```python
from build123d import *
from build123d.topology import SkipClean

# Parameters (mm, degrees)
CROQUIS1_R              = 25
SALIENTE_EXTRUIR1_DEPTH = 50
CORTAR_EXTRUIR1_DEPTH   = 50
MATRIZC2_COUNT          = 3
CROQUIS4_R              = 4
CROQUIS4_R_2            = 2
SALIENTE_EXTRUIR2_DEPTH = 15
CROQUIS4_2_R            = 2
CORTAR_EXTRUIR3_DEPTH   = 20
MATRIZC3_COUNT          = 3
MATRIZC4_COUNT          = 3
CROQUIS4_3_R            = 4
CROQUIS4_3_R_2          = 2
CORTAR_EXTRUIR4_DEPTH   = 2.5
MATRIZC5_COUNT          = 3


with BuildPart() as part:
    # Croquis1 → Saliente-Extruir1 (new body)
    with BuildSketch(Plane.XY):
        Circle(CROQUIS1_R)
    extrude(amount=SALIENTE_EXTRUIR1_DEPTH)

    # Croquis2 → Cortar-Extruir1 (cut)
    with BuildSketch(Plane(origin=(0, 0, 0), x_dir=(-1, 0, 0), z_dir=(0, 0, -1))):
        with BuildLine():
            Line((-15, 20), (15, 20))
            ThreePointArc((15, 20), (0, 25), (-15, 20))
        make_face()
    cortar_extruir1 = extrude(amount=-CORTAR_EXTRUIR1_DEPTH, mode=Mode.SUBTRACT)

    # MatrizC2: Cortar-Extruir1 ×3 about axis
    matrizc2_axis = Axis((0, 0, 0), (0, 0, 1))
    for i in range(1, MATRIZC2_COUNT):
        add(cortar_extruir1.rotate(matrizc2_axis, i * 360 / MATRIZC2_COUNT), mode=Mode.SUBTRACT)

    # Croquis4 → Saliente-Extruir2 (add, symmetric)
    with BuildSketch(Plane(origin=(0, 0, 0), x_dir=(0, 0, -1), z_dir=(1, 0, 0))):
        with Locations((0, 20)):
            Circle(CROQUIS4_R)
        with Locations((0, 20)):
            Circle(CROQUIS4_R_2, mode=Mode.SUBTRACT)
    saliente_extruir2 = extrude(amount=SALIENTE_EXTRUIR2_DEPTH, both=True)

    # Croquis4<2> → Cortar-Extruir3 (cut, symmetric)
    with SkipClean():  # the faces are left unmerged after this step: merging them gives an invalid solid
        with BuildSketch(Plane(origin=(0, 0, 0), x_dir=(0, 0, -1), z_dir=(1, 0, 0))):
            with Locations(Location((0, 20, 0), (0, 0, 180))):
                Circle(CROQUIS4_2_R)
        cortar_extruir3 = extrude(amount=CORTAR_EXTRUIR3_DEPTH, both=True, mode=Mode.SUBTRACT)

    # MatrizC3: Saliente-Extruir2 ×3 about axis
    with SkipClean():  # the faces are left unmerged after this step: merging them gives an invalid solid
        matrizc3_axis = Axis((0, 0, 0), (0, 0, 1))
        for i in range(1, MATRIZC3_COUNT):
            add(saliente_extruir2.rotate(matrizc3_axis, i * 360 / MATRIZC3_COUNT))

    # MatrizC4: Cortar-Extruir3 ×3 about axis
    with SkipClean():  # the faces are left unmerged after this step: merging them gives an invalid solid
        matrizc4_axis = Axis((0, 0, 50), (0, 0, -1))
        for i in range(1, MATRIZC4_COUNT):
            add(cortar_extruir3.rotate(matrizc4_axis, i * 360 / MATRIZC4_COUNT), mode=Mode.SUBTRACT)

    # Croquis4<3> → Cortar-Extruir4 (cut, symmetric)
    with BuildSketch(Plane(origin=(0, 0, 0), x_dir=(0, 0, -1), z_dir=(1, 0, 0))):
        with Locations((0, 20)):
            Circle(CROQUIS4_3_R)
        with Locations(Location((0, 20, 0), (0, 0, 180))):
            Circle(CROQUIS4_3_R_2, mode=Mode.SUBTRACT)
    cortar_extruir4 = extrude(amount=CORTAR_EXTRUIR4_DEPTH, both=True, mode=Mode.SUBTRACT)

    # MatrizC5: Cortar-Extruir4 ×3 about axis
    matrizc5_axis = Axis((0, 0, 0), (0, 0, 1))
    for i in range(1, MATRIZC5_COUNT):
        add(cortar_extruir4.rotate(matrizc5_axis, i * 360 / MATRIZC5_COUNT), mode=Mode.SUBTRACT)


solid = part.part
```
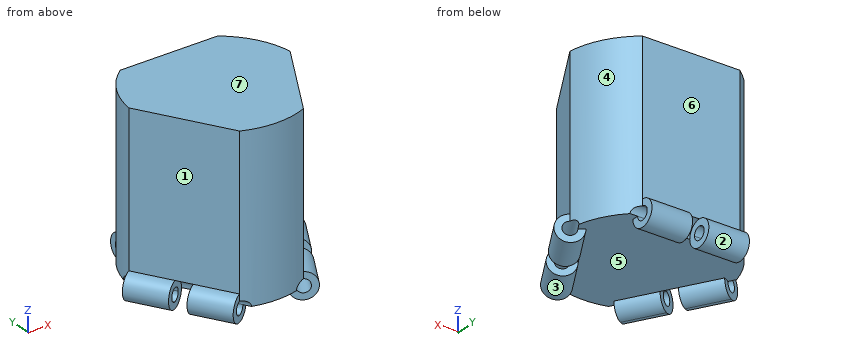
Build history of the part. All positions in model axes, mm. Face numbers are marked on the shaded views. A direction names the side the tool comes from. Round coordinates to 2 decimals unless told otherwise and drop trailing zeros. Order: outer loops, then holes, each group sorted by start corner. A loop starts at its lowest first (then second) coordinate and runs counter-clockwise, first axis right, second up. Notation, with made-up numbers: (-6.5, -30.5) -> (7.5, -30.5) arc R28 ccw to (7.5, 8.5) -> close; hole circle Ø7 at (-33, 64.5). An arc over 180 degrees is marked (long way). Answer in a Markdown table with one row per item.
1) Mould opens along X. For the marked faces 1, 2, 3 and 4 say: released by +X, released by -X, zero draft, split by the parting line, or undercut.
Values:
| item | result |
|---|---|
| face 1 | released by -X |
| face 2 | zero draft |
| face 3 | undercut |
| face 4 | released by +X |
2) Wall check: L1, parallel to Z at x = 1, y = -21.5; L2, parallel to X at y = 13, z = 30.5; L3, parallel to Y at x = 6, z = 27. Give the ranges that are in metal, low to high.
Values:
| item | result |
|---|---|
| L1 | 0 to 50 |
| L2 | -21.35 to 21.35 |
| L3 | -24.27 to 20 |
3) Band-saw the part on C-C on y = -2.5. Give the number of separate pieces and of enclosed holes in the cut face, and give its area (3 significant figures).
Values:
| item | result |
|---|---|
| separate pieces | 1 |
| enclosed holes | 2 |
| area | 2,220 mm2 |
4) Band-saw the part on A-A on z = 10. Give the cut face in (x, y), and give its area (3 significant figures).
Values:
| item | result |
|---|---|
| outline | (-24.82, 2.99) -> (-9.82, -22.99) arc R25 ccw to (9.82, -22.99) -> (24.82, 2.99) arc R25 ccw to (15, 20) -> (-15, 20) arc R25 ccw to start |
| area | 1,660 mm2 |
5) Which spindle directions (+Z, -Z, +X, -X, +Y, -Y) get a long thin tool onto all of the face, cutting with end or side? Do the marked faces 5, 6 and 7. Say none if no direction does.
Values:
| item | result |
|---|---|
| face 5 | -Z |
| face 6 | +Z, +X, -X, +Y |
| face 7 | +Z, +X, -X, +Y, -Y |
6) Pin check, flat tips, straight feed: P1, Ø9, axis at x = 3, z = 19.5, coming from the +Y side; P2, Ø5, axis at y = 20, z = 0, coming from the +X side; P3, Ø6, axis at x = 0.5, z = 16, coming from the -Y side. Stop position of each tip, or through.
Values:
| item | result |
|---|---|
| P1 | y = 20 |
| P2 | x = 17.85 |
| P3 | y = -25 |
7) Band-saw the part on B-B on y = 12.5. Give the cut face in (x, z), and give its area (3 significant figures).
Values:
| item | result |
|---|---|
| outline | (-21.65, 0) -> (21.65, 0) -> (21.65, 50) -> (-21.65, 50) -> close |
| area | 2,170 mm2 |
